Check sheet for the drawn part. Datum: minimum x, y, z corner. Units: mm. A direction names the side the tool comes from. Coordinates: 2 decimals unless noted, no trailing zeros. Loops run counter-clockwise (first coordinate to the right, second up) from the corner with the lowest first, then second, coordinate; pieces in that order, holes last.
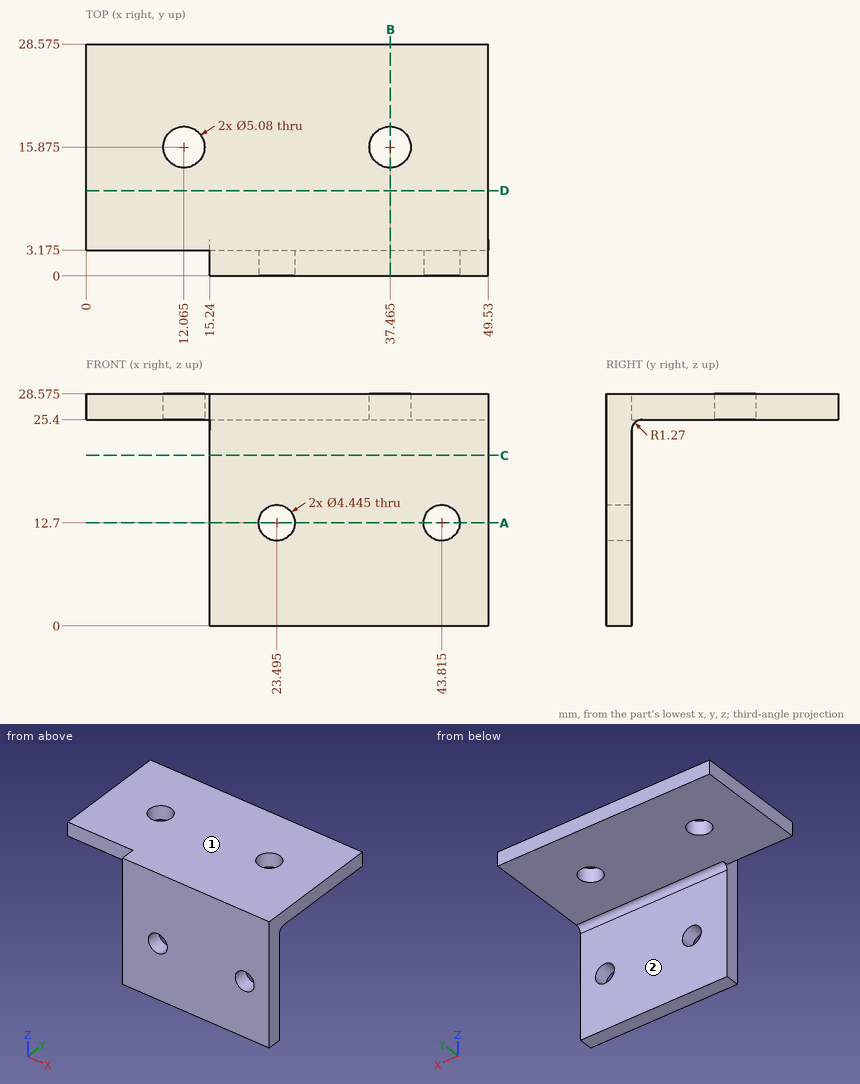
(1) Gauge pin test, flat ends, axial feed: pin 1 Ø12 at (x, z) = (24, 15.5) entering from +Y (3 decimals); pin 2 Ø3 at (x, y) = (23, 10.5) entering from -Z; pin 3 Ø10 at (x, z) = (37.5, 23) entering from -Y; pin 4 Ø4 at (x, y) = (37.465, 15.875) entering from -Z. Record the tip position at first contact, or that the pin passes through.
Findings:
pin 1: stops at y = 3.175
pin 2: stops at z = 25.4
pin 3: stops at y = 0
pin 4: passes through
(2) Scan lines: L1, parallel to X at y = 2.1, z = 12.7; L2, parallel to X at y = 14.5, z = 27; L3, parallel to Z at x = 31.5, y = 17.75 (3 decimals). Record each from-to range of solid material in increasing order.
Findings:
L1: x = 15.24 to 21.27, 25.72 to 41.59, 46.04 to 49.53
L2: x = 0 to 9.93, 14.2 to 35.33, 39.6 to 49.53
L3: z = 25.4 to 28.575
(3) Sectioned sample at A-A on z = 12.7. Record the cut outline in (x, y) (1 decimal), and give its area (3 significant figures).
Findings:
outline: (15.2, 0) - (21.3, 0) - (21.3, 3.2) - (15.2, 3.2) - close; (25.7, 0) - (41.6, 0) - (41.6, 3.2) - (25.7, 3.2) - close; (46, 0) - (49.5, 0) - (49.5, 3.2) - (46, 3.2) - close
area: 80.6 mm2
(4) Sectioned sample at C-C on z = 21. Record the cut outline in (x, y) (3 decimals).
Findings:
outline: (15.24, 0) - (49.53, 0) - (49.53, 3.175) - (15.24, 3.175) - close
(5) Access from +Z, -Z, +X, -X, +Y, -Y to the whole of each face (thin tool, end or side, straight path). Record for the marked faces 1 and 2.
Findings:
face 1: +Z, +X, -X, +Y, -Y
face 2: -Z, +X, -X, +Y
(6) Sectioned sample at B-B on x = 37.5. Record the cut outline in (y, z) (3 decimals).
Findings:
outline: (0, 0) - (3.175, 0) - (3.175, 24.13) arc R1.27 cw to (4.445, 25.4) - (13.335, 25.4) - (13.335, 28.575) - (0, 28.575) - close; (18.415, 25.4) - (28.575, 25.4) - (28.575, 28.575) - (18.415, 28.575) - close
(7) Sectioned sample at D-D on y = 10.5. Record the cut outline in (x, z) (3 decimals).
Findings:
outline: (0, 25.4) - (49.53, 25.4) - (49.53, 28.575) - (0, 28.575) - close
